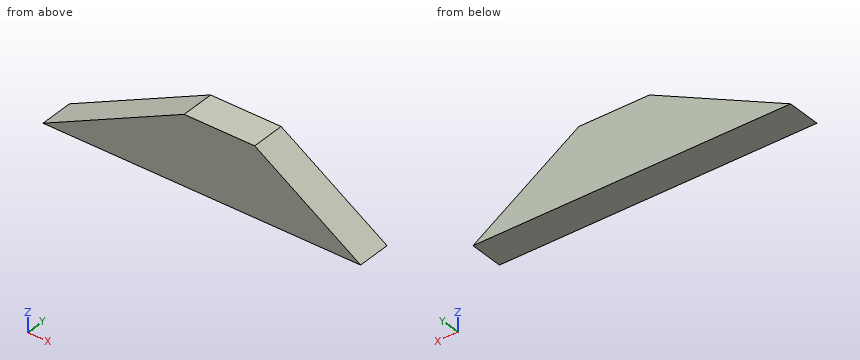
from build123d import *

# Parameters (mm, degrees)
F0_W     = 100
F0_H     = 98
F1_DEPTH = 48


# Not quite as in the source:
# - a feature names something its author has since deleted; it is built from what else it names


with BuildPart() as f1:
    # F0 (on Front) → F1 (new body)
    with BuildSketch(Plane.XZ):
        Rectangle(F0_W, F0_H)
        Polygon((-250, -49), (-50, -49), (-50, 49), (-50, 49.0569584072), align=None)
        Polygon((50, 49), (50, -49), (200, -49), (50, 49.0569546819), align=None)
    extrude(amount=F1_DEPTH)


solid = f1.part
Design review of the part built by this model. Coordinates are the model's own, in mm. Coordinates: 2 decimals unless noted, no trailing zeros. Order: outer loops, then holes, each group sorted by start corner. A loop starts at its lowest first (then second) coordinate and runs counter-clockwise, first axis right, second up. Notation, with made-up numbers: (48.25, -25.75) - (75.25, -25.75) arc R27 ccw to (75.25, 2.25) - close; hole circle Ø11 at (-35.75, -37.5). An arc over 180 degrees is marked (long way). Put each result on its own line as item: value.
1) Wall thickness on L1, parallel to Z at x = -43, y = -42; L2, parallel to X at y = -20, z = 21; L3, parallel to Z at x = -169, y = -2: over which ranges is each line inside the solid? List them lowest first. Write a range as from..to.
Response values:
L1: z = -49..49
L2: x = -107.23..92.92
L3: z = -49..-9.29
2) Take a section at A-A, the plane y = -4.5. Give the boundary of the cut face in (x, z), and give its area (3 significant figures).
Response values:
outline: (-250, -49) - (200, -49) - (50, 49.06) - (50, 49) - (-50, 49) - (-50, 49.06) - close
area: 27,000 mm²
3) Take a section at B-B, the plane z = -22. Give the boundary of the cut face in (x, y), and give its area (3 significant figures).
Response values:
outline: (-194.93, -48) - (158.7, -48) - (158.7, 0) - (-194.93, 0) - close
area: 17,000 mm²
4) Take a section at C-C, the plane x = -74.5. Give the boundary of the cut face in (y, z).
Response values:
outline: (-48, -49) - (0, -49) - (0, 37.04) - (-48, 37.04) - close
5) Insertion check: P1, Ø6, axis at y = -6, z = 28, coming from the -X side; P2, Ø12, axis at y = -25, z = 17, coming from the -X side; P3, Ø1.5, axis at x = 18.5, y = -43, coming from the +Z side. Each pin has a flat end and moves straight along its axis. Give the tip position at first contact, or say it passes through.
Response values:
P1: stops at x = -99.07
P2: stops at x = -127.62
P3: stops at z = 49
